from build123d import *

# Parameters (mm, degrees)
SKETCH_1_W          = 67
SKETCH_1_H          = 41
EXTRUDE_1_DEPTH     = 6.5
SKETCH_2_W          = 64
SKETCH_2_H          = 38
CUT_EXTRUDE_1_DEPTH = 4.5
FILLET_1_R          = 1
FILLET_2_R          = 2
SKETCH_3_R          = 3
EXTRUDE_2_DEPTH     = 3
SKETCH_4_R          = 1.5
CUT_EXTRUDE_2_DEPTH = 6
CHAMFER_1_SIZE      = 3
CHAMFER_2_SIZE      = 2


with BuildPart() as part:
    # Эскиз1 → Бобышка-Вытянуть1 (new body)
    with BuildSketch(Plane(origin=(0, 0, 0), x_dir=(1, 0, 0), z_dir=(0, 1, 0))):
        Rectangle(SKETCH_1_W, SKETCH_1_H)
    extrude(amount=EXTRUDE_1_DEPTH)

    # Эскиз2 → Вырез-Вытянуть1 (cut)
    with BuildSketch(Plane(origin=(0, 6.5, 0), x_dir=(1, 0, 0), z_dir=(0, 1, 0))):
        Rectangle(SKETCH_2_W, SKETCH_2_H)
    extrude(amount=-CUT_EXTRUDE_1_DEPTH, mode=Mode.SUBTRACT)

    # Скругление1
    fillet_1_edges = [part.edges().sort_by_distance(p)[0] for p in [
        (32, 4.25, -19),
        (32, 4.25, 19),
        (-32, 4.25, 19),
        (-32, 4.25, -19),
    ]]
    fillet(fillet_1_edges, radius=FILLET_1_R)

    # Скругление2
    fillet_2_edges = [part.edges().sort_by_distance(p)[0] for p in [
        (33.5, 3.25, 20.5),
        (-33.5, 3.25, 20.5),
        (-33.5, 3.25, -20.5),
        (33.5, 3.25, -20.5),
    ]]
    fillet(fillet_2_edges, radius=FILLET_2_R)

    # Эскиз3 → Бобышка-Вытянуть2 (add)
    with BuildSketch(Plane(origin=(0, 2, 0), x_dir=(1, 0, 0), z_dir=(0, 1, 0))):
        with Locations(Location((28.6, 15.4, 0), (0, 0, 270))):
            Circle(SKETCH_3_R)
        with Locations(Location((4, 15.4, 0), (0, 0, 270))):
            Circle(SKETCH_3_R)
        with Locations(Location((4, -15.4, 0), (0, 0, 270))):
            Circle(SKETCH_3_R)
        with Locations(Location((28.6, -15.4, 0), (0, 0, 270))):
            Circle(SKETCH_3_R)
    extrude(amount=EXTRUDE_2_DEPTH)

    # Эскиз4 → Вырез-Вытянуть2 (cut)
    with BuildSketch(Plane(origin=(0, 5, 0), x_dir=(1, 0, 0), z_dir=(0, 1, 0))):
        with Locations(Location((4, 15.4, 0), (0, 0, 270))):
            Circle(SKETCH_4_R)
        with Locations(Location((28.6, 15.4, 0), (0, 0, 270))):
            Circle(SKETCH_4_R)
        with Locations(Location((28.6, -15.4, 0), (0, 0, 270))):
            Circle(SKETCH_4_R)
        with Locations(Location((4, -15.4, 0), (0, 0, 270))):
            Circle(SKETCH_4_R)
    extrude(amount=-CUT_EXTRUDE_2_DEPTH, mode=Mode.SUBTRACT)

    # Фаска1
    chamfer_1_edges = [part.edges().sort_by_distance(p)[0] for p in [
        (28.6, 0, -16.9),
        (4, 0, -16.9),
        (4, 0, 13.9),
        (28.6, 0, 13.9),
    ]]
    chamfer(chamfer_1_edges, length=CHAMFER_1_SIZE)

    # Фаска2
    # the kernel refuses this chamfer: 2 mm, written as the material it adds along each edge
    with BuildSketch(Plane(origin=(28.6, 2, -15.4), x_dir=(0, 0, 1), z_dir=(-1, 0, 0))) as chamfer_2_piece_1_section:
        Polygon((3, CHAMFER_2_SIZE), (3 + CHAMFER_2_SIZE, 0), (3, 0), align=None)
    chamfer_2_piece_1 = revolve(axis=Axis((28.6, 2, -15.4), (0, 1, 0)), mode=Mode.PRIVATE)
    chamfer_2_piece_1 = split(chamfer_2_piece_1, bisect_by=Plane(origin=(32, 3.643767664, -12.314318949), z_dir=(-1, 0, 0)), keep=Keep.TOP, mode=Mode.PRIVATE)
    add(chamfer_2_piece_1)
    with BuildSketch(Plane(origin=(4, 2, -15.4), x_dir=(0, 0, 1), z_dir=(-1, 0, 0))) as chamfer_2_piece_2:
        Polygon((3 + CHAMFER_2_SIZE, 0), (3, CHAMFER_2_SIZE), (3, 0), align=None)
    revolve(axis=Axis((4, 2, -15.4), (0, 1, 0)))
    with BuildSketch(Plane(origin=(28.6, 2, 15.4), x_dir=(0, 0, 1), z_dir=(-1, 0, 0))) as chamfer_2_piece_3_section:
        Polygon((3 + CHAMFER_2_SIZE, 0), (3, CHAMFER_2_SIZE), (3, 0), align=None)
    chamfer_2_piece_3 = revolve(axis=Axis((28.6, 2, 15.4), (0, 1, 0)), mode=Mode.PRIVATE)
    chamfer_2_piece_3 = split(chamfer_2_piece_3, bisect_by=Plane(origin=(32, 3.313770234, 18.884228213), z_dir=(-1, 0, 0)), keep=Keep.TOP, mode=Mode.PRIVATE)
    add(chamfer_2_piece_3)
    with BuildSketch(Plane(origin=(4, 2, 15.4), x_dir=(0, 0, 1), z_dir=(-1, 0, 0))) as chamfer_2_piece_4:
        Polygon((3 + CHAMFER_2_SIZE, 0), (3, CHAMFER_2_SIZE), (3, 0), align=None)
    revolve(axis=Axis((4, 2, 15.4), (0, 1, 0)))


solid = part.part
Input: part model. Units: mm. Frame: model coordinates. A direction names the side the tool comes from. Round coordinates to 2 decimals unless told otherwise and drop trailing zeros. Write each loop counter-clockwise with the first axis right and the second up, starting at its lowest first coordinate (ties: lowest second). Pieces come first, ordered by that corner, then holes.
1) Reachability of faces 4 (the cylindrical face through (32.9, 3.3, 19.93)), 5 (the flat face through (-32, 4, 0)) from +Z, -Z, +X, -X, +Y, -Y: full face, straight path, thin tool, end or side. Return the list, or none.
2) Cut plane C-C (x = 18.5). Return the cut outline in (y, z), then the cut area to 3 significant figures.
3) Cut plane D-D (z = -8.5). Return the cut outline in (x, y), then the cut area to 4 significant figures.
4) Ray query, L1, parallel to X at y = 4.45, z = -15.4; L2, parallel to Z at x = 10, y = 2.25; L3, parallel to X at y = 4.5, z = -18. Return the intervals inside material, ascending.
5) Cut plane A-A (x = 4). Count the separate pieces of the cut face and the enclosed holes in it, then the cut area to 3 significant figures.
6) Contact query for flat-ended pins moving along their axis: P1, Ø11.5, axis at x = 4, z = 6.5, coming from the +Y side; P2, Ø3, axis at x = 29.5, z = 14.5, coming from the +Y side. Output: stop coordinate, or through.
7) Draft query along X for faces 1 (the flat face through (0, 0, 0)), 2 (the flat face through (-33.5, 3, 0)), 3 (the cylindrical face through (25.67, 4.49, -16.05)). Return one class per face: pulls with the +X half, pulls with the -X half, needs draft (parallel to the pull), parting line crosses it, or undercut.
Geometry says:
1. face 4: +Z, +X, +Y, -Y
1. face 5: +Y
2. outline: (0, -20.5) - (6.5, -20.5) - (6.5, -19) - (2, -19) - (2, 19) - (6.5, 19) - (6.5, 20.5) - (0, 20.5) - close
2. area: 95.5 mm2
3. outline: (-33.5, 0) - (33.5, 0) - (33.5, 6.5) - (32, 6.5) - (32, 2) - (-32, 2) - (-32, 6.5) - (-33.5, 6.5) - close
3. area: 147.5 mm2
4. L1: x = -33.5 to -32, 1 to 2.5, 5.5 to 7, 25.6 to 27.1, 30.1 to 31.6, 32 to 33.5
4. L2: z = -20.5 to -19, 19 to 20.5
4. L3: x = -33.5 to -32, 2.5 to 5.5, 27.1 to 30.1, 32 to 33.5
5. separate pieces: 3
5. enclosed holes: 0
5. area: 89.5 mm2
6. P1: stops at y = 3.85
6. P2: stops at y = 5
7. face 1: needs draft
7. face 2: pulls with the -X half
7. face 3: undercut
